Geometry check sheet. Reference: the model listing, model coordinates, mm. A direction names the side the tool comes from. Round coordinates to 2 decimals unless told otherwise and drop trailing zeros. Order: outer loops, then holes, each group sorted by start corner. A loop starts at its lowest first (then second) coordinate and runs counter-clockwise, first axis right, second up. Notation, with made-up numbers: (66.25, 48) -> (115.25, 48) arc R34 cw to (115.25, 87) -> close; hole circle Ø3 at (-13, 3). An arc over 180 degrees is marked (long way). Use a Markdown table: item, result. Add a question column.
Item 1: Gauge pin test, flat ends, axial feed: pin 1 Ø4 at (y, z) = (-3.5, 5) entering from -X; pin 2 Ø2 at (x, y) = (14, 6.5) entering from +Z; pin 3 Ø2 at (x, z) = (4.5, -5.5) entering from -Y; pin 4 Ø10 at (x, y) = (7.5, -1) entering from -Z. Record the tip position at first contact, or that the pin passes through.
Item 2: Sectioned sample at C-C, the plane z = 1.25. Record the cut outline in (x, y), and give its area (3 significant figures).
Item 3: Material ranges on probe 1 along Y at (x, z) = (8, -0.25); probe 2 along Y at (x, z) = (8, -4.5); probe 3 along X at (y, z) = (0, -3.25), recorded low to high. Write a range as [from, to].
Item 4: Set-up check for faces 4 (the cylindrical face through (10.575, 0.811, 0.72)), 5 (the cylindrical face through (3.32, 2.98, 3.15)), 6 (the cylindrical face through (1.12, -0.65, -2.93)), 7 (the flat face through (4.26, -1.42, -2.08)): record each of +Z, -Z, +X, -X, +Y, -Y from which the full face is reachable in a straight line by a thin tool's end or side.
Item 5: Sectioned sample at D-D, the plane x = 2. State how many separate pieces and enclosed holes the cut face has, and give its area (3 significant figures).
Item 6: Mould release check, pull along Z, two halves, no side actions. Record for faces 1 (the flat face through (12, 0, -8)), 2 (the flat face through (5.5, 2, -5)), 3 (the conical face through (13.598, -1.243, -0.346)): pulls with the +Z half, pulls with the -Z half, needs draft (parallel to the pull), parting line crosses it, or undercut.
Item 7: Sectioned sample at B-B, the plane z = -5. Record the cut outline in (x, y).
Item 8: Sectioned sample at A-A, the plane x = 8. Record the cut outline in (y, z), and give its area (3 significant figures).
from build123d import *

# Parameters (mm, degrees)
BORE_START          = 1
SKETCH_2_R          = 2.7
BORE_DEPTH          = 19.2
FIX_START           = 3.2
SKETCH_4_R          = 1.7
FIX_2_DEPTH         = 6.3
CUT_EXTRUDE_START   = 2.5
SKETCH_4_3_R        = 1.7
CUT_EXTRUDE_1_DEPTH = 2.8
MOVE_BODY_1_ANGLE   = 90
FILLET_1_R          = 0.15


with BuildPart() as part:
    # Sketch 1 → Body (revolve)
    with BuildSketch(Plane.XY):
        with BuildLine():
            Line((0, 8.5), (0, 0))
            Line((0, 0), (17.2, 0))
            Line((17.2, 0), (17.2, 3.958583851))
            Line((17.2, 3.958583851), (16.652924896, 5.61704678))
            ThreePointArc((16.652924896, 5.61704678), (15.650028154, 6.31642018), (14.697387016, 5.55))
            Line((14.697387016, 5.55), (7.697387016, 5.55))
            Line((7.697387016, 5.55), (7, 8.5))
            Line((7, 8.5), (0, 8.5))
        make_face()
    revolve(axis=Axis((0, 0, 0), (1, 0, 0)))

    # Sketch 2 → Bore (cut, through all)
    with BuildSketch(Plane(origin=(17.2, 0, 0), x_dir=(0, 0, -1), z_dir=(1, 0, 0)).offset(BORE_START)):
        Circle(SKETCH_2_R)
    extrude(amount=-BORE_DEPTH, mode=Mode.SUBTRACT)

    # Sketch 4 → Fix 2 (cut, through all)
    with BuildSketch(Plane.XY.offset(FIX_START)):
        with Locations((3.5, 0)):
            Circle(SKETCH_4_R)
    extrude(amount=FIX_2_DEPTH, mode=Mode.SUBTRACT)

    # Sketch 4_3 → Cut-Extrude 1 (cut)
    with BuildSketch(Plane.XY.offset(CUT_EXTRUDE_START)):
        Polygon((-1.112463997, 2.806157241), (-1.112463997, -2.806157241), (1.825684219, -2.806157241), (5.120135639, -2.806157241), (6.740271277, 0), (5.120135639, 2.806157241), (1.825684219, 2.806157241), align=None)
        with Locations((3.5, 0)):
            Circle(SKETCH_4_3_R, mode=Mode.SUBTRACT)
        with Locations((3.5, 0)):
            Circle(SKETCH_4_3_R)
    extrude(amount=CUT_EXTRUDE_1_DEPTH, mode=Mode.SUBTRACT)


with BuildPart() as part_1:
    # Move Body 1: moved
    add(part.part.rotate(Axis((8, 0, 0), (0, -1, 0)), MOVE_BODY_1_ANGLE))

    # Fillet 1
    fillet_1_edges = [part_1.edges().sort_by_distance(p)[0] for p in [
        (5.5, 1.019803903, -4.92425639),
        (5.5, -1.019803903, -4.92425639),
    ]]
    fillet(fillet_1_edges, radius=FILLET_1_R)


solid = part_1.part
Found:
| question | item | result |
|---|---|---|
| 1 | pin 1 | stops at x = 2.66 |
| 1 | pin 2 | stops at z = -0.85 |
| 1 | pin 3 | stops at y = -8.12 |
| 1 | pin 4 | stops at z = -8 |
| 2 | outline | circle Ø11.1 at (8, 0); hole circle Ø5.4 at (8, 0) |
| 2 | area | 73.9 mm2 |
| 3 | probe 1 | y = [-5.55, -2.7], [2.7, 5.55] |
| 3 | probe 2 | y = [-8.5, -2.7], [2.7, 8.5] |
| 3 | probe 3 | x = [10.7, 16.5] |
| 4 | face 4 | +Z, -Z |
| 4 | face 5 | none |
| 4 | face 6 | -X |
| 4 | face 7 | -Z |
| 5 | separate pieces | 2 |
| 5 | enclosed holes | 1 |
| 5 | area | 84.5 mm2 |
| 6 | face 1 | pulls with the -Z half |
| 6 | face 2 | needs draft |
| 6 | face 3 | undercut |
| 7 | outline | (-0.34, -1.62) arc R8.5 ccw (long way) to (-0.34, 1.62) -> (2.7, 1.62) -> (2.7, 2.81) -> (5.5, 2.81) -> (5.5, 1.61) arc R0.15 ccw to (5.77, 1.53) arc R2.7 cw (long way) to (5.77, -1.53) arc R0.15 ccw to (5.5, -1.61) -> (5.5, -2.81) -> (2.7, -2.81) -> (2.7, -1.62) -> close |
| 8 | outline | (-8.5, -8) -> (-2.7, -8) -> (-2.7, 9.2) -> (-3.96, 9.2) -> (-5.62, 8.65) arc R1.02 ccw to (-5.55, 6.7) -> (-5.55, -0.3) -> (-8.5, -1) -> close; (2.7, -8) -> (8.5, -8) -> (8.5, -1) -> (5.55, -0.3) -> (5.55, 6.7) arc R1.02 ccw to (5.62, 8.65) -> (3.96, 9.2) -> (2.7, 9.2) -> close |
| 8 | area | 143 mm2 |
